from build123d import *

# Parameters (mm, degrees)
STATOR_ENVELOPE_START     = -53.3
PROFILE_1_R               = 28.5
PROFILE_1_R_2             = 1.25
STATOR_ENVELOPE_DEPTH     = 52.3
ROTOR_REVIEW_RECESS_START = -5.2
PROFILE_2_R               = 17.65
ROTOR_REVIEW_RECESS_DEPTH = 4.3


with BuildPart() as part:
    # Profile_1 → Stator_envelope (new body)
    with BuildSketch(Plane.XY.offset(STATOR_ENVELOPE_START)):
        Circle(PROFILE_1_R)
        with Locations((21.650635095, 12.5)):
            Circle(PROFILE_1_R_2, mode=Mode.SUBTRACT)
        with Locations((0, 25)):
            Circle(PROFILE_1_R_2, mode=Mode.SUBTRACT)
        with Locations((-21.650635095, 12.5)):
            Circle(PROFILE_1_R_2, mode=Mode.SUBTRACT)
        with Locations((-21.650635095, -12.5)):
            Circle(PROFILE_1_R_2, mode=Mode.SUBTRACT)
        with Locations((0, -25)):
            Circle(PROFILE_1_R_2, mode=Mode.SUBTRACT)
        with Locations((21.650635095, -12.5)):
            Circle(PROFILE_1_R_2, mode=Mode.SUBTRACT)
    extrude(amount=STATOR_ENVELOPE_DEPTH)

    # Profile_2 → Rotor_review_recess (cut)
    with BuildSketch(Plane.XY.offset(ROTOR_REVIEW_RECESS_START)):
        with Locations(Location((0, 0, 0), (0, 0, 180))):
            Circle(PROFILE_2_R)
    extrude(amount=ROTOR_REVIEW_RECESS_DEPTH, mode=Mode.SUBTRACT)


solid = part.part
CAD build for the part. Positions are in the model's coordinates, mm. A direction names the side the tool comes from. Coordinates: 2 decimals unless noted, no trailing zeros. Loops run counter-clockwise (first coordinate to the right, second up) from the corner with the lowest first, then second, coordinate; pieces in that order, holes last. Notation, with made-up numbers: (-27.75, -28) - (-6.75, -28) arc R26 ccw to (-6.75, 10) - close; hole circle Ø5 at (9, 61). An arc over 180 degrees is marked (long way). Write item = value, one per line. Start each with the question number.
Q1. Cut at D-D, the plane y = 25. List the corners of the cut face in (x, z).
Q2. Cut at B-B, the plane x = 0. List the corners of the cut face in (y, z), then the cut area to 3 significant figures.
Q3. Which spindle directions (+Z, -Z, +X, -X, +Y, -Y) get a long thin tool onto all of the face, cutting with end or side? Do faces 4 (the flat face through (0, 0, -5.2)), 5 (the cylindrical face through (-0.27, 23.78, -27.52)). Say none if no direction does.
Q4. Cut at C-C, the plane z = -29. List the corners of the cut face in (x, y).
Q5. Drill centre lines: L1, parallel to Y at x = 0, z = -33; L2, parallel to X at y = -13.5, z = -36; L3, parallel to Y at x = 0.5, z = -50. Where is each one in solid material? Low to high.
Q6. Pull direction Y, two halves, no side cores. Call faces 1 (the cylindrical face through (22.323, -11.446, -27.516)), 2 (the cylindrical face through (26.327, -10.916, -27.516)), 3 (the flat face through (-13.1, -12.3, -1)): pulls with the +Y half, pulls with the -Y half, needs draft (parallel to the pull), parting line crosses it, or undercut.
Q7. Cut at A-A, the plane y = 0. List the corners of the cut face in (x, z), then the cut area to 3 significant figures.
Q8. Flat gauge pins, fed straight in: pin 1 Ø5 at (y, z) = (-13.5, -47.5) entering from +X; pin 2 Ø4 at (y, z) = (22, -22) entering from -X; pin 3 Ø3 at (x, y) = (21.65, -12.5) entering from -Z; pin 4 Ø2 at (x, y) = (21.65, 12.5) entering from -Z. Where does each tip first touch, or does it go through?
Computed:
q1.outline = (-13.68, -53.3) - (-1.25, -53.3) - (-1.25, -1) - (-13.68, -1) - close; (1.25, -53.3) - (13.68, -53.3) - (13.68, -1) - (1.25, -1) - close
q2.outline = (-28.5, -53.3) - (-26.25, -53.3) - (-26.25, -1) - (-28.5, -1) - close; (-23.75, -53.3) - (23.75, -53.3) - (23.75, -1) - (17.65, -1) - (17.65, -5.2) - (-17.65, -5.2) - (-17.65, -1) - (-23.75, -1) - close; (26.25, -53.3) - (28.5, -53.3) - (28.5, -1) - (26.25, -1) - close
q2.area = 2,570 mm²
q3.face_4 = +Z
q3.face_5 = +Z, -Z
q4.outline = circle Ø57 at (0, 0); hole circle Ø2.5 at (-21.65, -12.5); hole circle Ø2.5 at (-21.65, 12.5); hole circle Ø2.5 at (0, -25); hole circle Ø2.5 at (0, 25); hole circle Ø2.5 at (21.65, -12.5); hole circle Ø2.5 at (21.65, 12.5)
q5.L1 = -28.5 to -26.25, -23.75 to 23.75, 26.25 to 28.5
q5.L2 = -25.1 to -22.4, -20.9 to 20.9, 22.4 to 25.1
q5.L3 = -28.5 to -26.15, -23.85 to 23.85, 26.15 to 28.5
q6.face_1 = undercut
q6.face_2 = parting line crosses it
q6.face_3 = needs draft
q7.outline = (-28.5, -53.3) - (28.5, -53.3) - (28.5, -1) - (17.65, -1) - (17.65, -5.2) - (-17.65, -5.2) - (-17.65, -1) - (-28.5, -1) - close
q7.area = 2,830 mm²
q8.pin_1 = 26.29
q8.pin_2 = -20.3
q8.pin_3 = -53.3
q8.pin_4 = through
